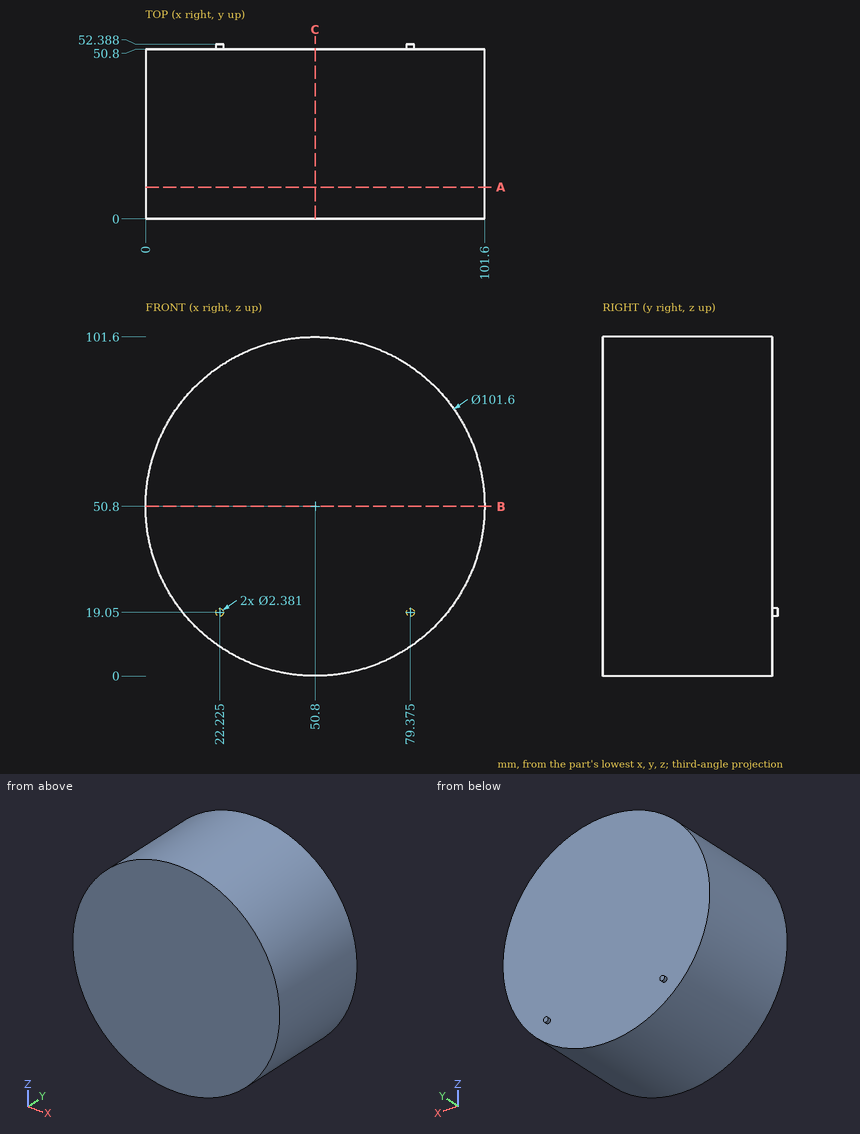
Design review of the part shown in the three views and the two pictorial views. Dimensions are in mm from the part's minimum x, y and z. Round coordinates to 2 decimals unless told otherwise and drop trailing zeros. Loops run counter-clockwise (first coordinate to the right, second up) from the corner with the lowest first, then second, coordinate; pieces in that order, holes last.
1) Consider section A-A on y = 9.5. State the section outline as (x, z) points.
Values follow:
outline: circle Ø101.6 at (50.8, 50.8)
2) Consider section B-B on z = 50.8. State the section outline as (x, y) points, then the cut area to 3 significant figures.
Values follow:
outline: (0, 0) - (101.6, 0) - (101.6, 50.8) - (0, 50.8) - close
area: 5,160 mm2
3) Clearance check with flat-ended pins moving along their axes: P1, Ø3, axis at x = 18, z = 40, coming from the +Y side; P2, Ø8, axis at y = 26.5, z = 84, coming from the -X side; P3, Ø1.5, axis at x = 18, y = 17.5, coming from the +Z side; P4, Ø1.5, axis at x = 69, z = 19.5, coming from the -Y side. State where each tip first meets the part, or that it passes through.
Values follow:
P1: stops at y = 50.8
P2: stops at x = 9.23
P3: stops at z = 90.21
P4: stops at y = 0
4) Wall thickness on line 1 along Y through (x, z) = (20, 72.5); line 2 along X through (y, z) = (6.5, 65.5); line 3 along X through (y, z) = (16, 78.5): over which ranges is each line inside the solid? List them lowest first.
Values follow:
line 1: y = 0 to 50.8
line 2: x = 2.17 to 99.43
line 3: x = 8.22 to 93.38
5) Consider section C-C on x = 50.8. State the section outline as (y, z) points, then the cut area to 3 significant figures.
Values follow:
outline: (0, 0) - (50.8, 0) - (50.8, 101.6) - (0, 101.6) - close
area: 5,160 mm2
